Geometry check sheet. Reference: the model listing, model coordinates, mm. A direction names the side the tool comes from. Round coordinates to 2 decimals unless told otherwise and drop trailing zeros. Loops run counter-clockwise (first coordinate to the right, second up) from the corner with the lowest first, then second, coordinate; pieces in that order, holes last. Notation, with made-up numbers: (74, -35) -> (124, -35) arc R29 cw to (124, -11) -> close; hole circle Ø6 at (77, 71.25). An arc over 180 degrees is marked (long way). Use one line per item in the form item = value.
from build123d import *

# Parameters (mm, degrees)
BOSS_EXTRUDE1_DEPTH     = 12
CUT_EXTRUDE1_DEPTH      = 35.812889373272625
CUT_EXTRUDE1_DEPTH_BACK = 35.812889373272625
BOSS_EXTRUDE2_DEPTH     = 8
CUT_EXTRUDE2_DEPTH      = 2.5
CUT_EXTRUDE3_DEPTH      = 5
SKETCH8_R               = 1.4999999999999996
BOSS_EXTRUDE3_DEPTH     = 5.499999999999998
CUT_EXTRUDE4_DEPTH      = 35.812889373272625
CUT_EXTRUDE4_DEPTH_BACK = 35.812889373272625
SKETCH9_W               = 12
SKETCH9_H               = 6.684402113618233
CUT_EXTRUDE5_DEPTH      = 1


with BuildPart() as part:
    # Sketch1 → Boss-Extrude1 (new body)
    with BuildSketch(Plane.XY):
        with BuildLine():
            Line((-56.57427779976257, 0), (-40.22081023433309, 0))
            Line((-40.22081023433309, 0), (-41.713141903429594, 24.955419174788705))
            ThreePointArc((-41.713141903429594, 24.955419174788705), (-48.397544017047835, 31.639821288406946), (-55.081946130666076, 24.955419174788705))
            Line((-55.081946130666076, 24.955419174788705), (-56.57427779976257, 0))
        make_face()
    extrude(amount=BOSS_EXTRUDE1_DEPTH)

    # Sketch3 → Cut-Extrude1 (cut, two sides: drawn at the far end of the back side and taken through both)
    with BuildSketch(Plane(origin=(-48.39754401704783, 0, 0), x_dir=(0, 0, -1), z_dir=(1, 0, 0)).offset(-CUT_EXTRUDE1_DEPTH_BACK)):
        Polygon((-12, 6.613954943904592), (-12, 0), (-4, -4.9e-16), align=None)
    extrude(amount=CUT_EXTRUDE1_DEPTH + CUT_EXTRUDE1_DEPTH_BACK, mode=Mode.SUBTRACT)

    # Sketch6 → Boss-Extrude2 (add, symmetric)
    with BuildSketch(Plane(origin=(-48.39754401704783, 0, 0), x_dir=(0, 0, -1), z_dir=(1, 0, 0))):
        with BuildLine():
            ThreePointArc((-2.9999999999999982, -1.1000000000000008), (-3.0526985696936526, -0.5401658469562882), (-3.2089428526094457, 4.952e-14))
            Line((-3.2089428526094603, 0), (-4.98019609728148, 0))
            ThreePointArc((-4.980196097281471, 2.665e-14), (-4.62528078247269, -0.499877451714149), (-4.499999999999998, -1.1000000000000008))
            ThreePointArc((-4.499999999999998, -1.1000000000000012), (-6.600122548285821, -2.474719217527322), (-7.0198039027185715, -1.621e-14))
            Line((-7.019803902718577, 0), (-8.7910571473906, 0))
            ThreePointArc((-8.791057147390587, -4.152e-14), (-6.5598341530436635, -4.047301430306355), (-2.9999999999999982, -1.1000000000000014))
        make_face()
        with BuildLine():
            Line((-4.98019609728148, 0), (-3.2089428526094603, 0))
            ThreePointArc((-3.2089428526094457, 4.952e-14), (-6.000000000000047, 1.8999999999999992), (-8.791057147390587, -4.152e-14))
            Line((-8.7910571473906, 0), (-7.019803902718577, 0))
            ThreePointArc((-7.0198039027185715, -1.621e-14), (-6.00000000000003, 0.3999999999999988), (-4.980196097281471, 2.665e-14))
        make_face()
    extrude(amount=BOSS_EXTRUDE2_DEPTH, both=True)

    # Sketch6_3 → Cut-Extrude2 (cut, symmetric)
    with BuildSketch(Plane(origin=(-48.39754401704783, 0, 0), x_dir=(0, 0, -1), z_dir=(1, 0, 0))):
        with BuildLine():
            ThreePointArc((-2.9999999999999982, -1.1000000000000008), (-3.0526985696936526, -0.5401658469562882), (-3.2089428526094457, 4.952e-14))
            Line((-3.2089428526094603, 0), (-4.98019609728148, 0))
            ThreePointArc((-4.980196097281471, 2.665e-14), (-4.62528078247269, -0.499877451714149), (-4.499999999999998, -1.1000000000000008))
            ThreePointArc((-4.499999999999998, -1.1000000000000012), (-6.600122548285821, -2.474719217527322), (-7.0198039027185715, -1.621e-14))
            Line((-7.019803902718577, 0), (-8.7910571473906, 0))
            ThreePointArc((-8.791057147390587, -4.152e-14), (-6.5598341530436635, -4.047301430306355), (-2.9999999999999982, -1.1000000000000014))
        make_face()
        with BuildLine():
            Line((-4.98019609728148, 0), (-3.2089428526094603, 0))
            ThreePointArc((-3.2089428526094457, 4.952e-14), (-6.000000000000047, 1.8999999999999992), (-8.791057147390587, -4.152e-14))
            Line((-8.7910571473906, 0), (-7.019803902718577, 0))
            ThreePointArc((-7.0198039027185715, -1.621e-14), (-6.00000000000003, 0.3999999999999988), (-4.980196097281471, 2.665e-14))
        make_face()
    extrude(amount=CUT_EXTRUDE2_DEPTH, both=True, mode=Mode.SUBTRACT)

    # Sketch7 → Cut-Extrude3 (cut, symmetric)
    with BuildSketch(Plane(origin=(-48.39754401704783, 0, 0), x_dir=(0, 0, -1), z_dir=(1, 0, 0))):
        Polygon((-7.161655697006073, 2.6138810410171796), (-11.015220244212237, 5.799793827098392), (-7.829307458131025, 9.653358374304556), (-3.9757429109248625, 6.467445588223342), align=None)
    extrude(amount=CUT_EXTRUDE3_DEPTH, both=True, mode=Mode.SUBTRACT)

    # Sketch8 → Boss-Extrude3 (add, symmetric)
    with BuildSketch(Plane(origin=(-48.39754401704783, 0, 0), x_dir=(0, 0, -1), z_dir=(1, 0, 0))):
        with Locations((-7.548090255966457, 6.177113636233633)):
            Circle(SKETCH8_R)
    extrude(amount=BOSS_EXTRUDE3_DEPTH, both=True)

    # Sketch9 → Cut-Extrude4 (cut, two sides: drawn at the far end of the back side and taken through both)
    with BuildSketch(Plane(origin=(-48.39754401704783, 0, 0), x_dir=(0, 0, -1), z_dir=(1, 0, 0)).offset(-CUT_EXTRUDE4_DEPTH_BACK)):
        with Locations((-6, 28.297620231597822)):
            Rectangle(SKETCH9_W, SKETCH9_H)
    extrude(amount=CUT_EXTRUDE4_DEPTH + CUT_EXTRUDE4_DEPTH_BACK, mode=Mode.SUBTRACT)

    # Sketch10 → Cut-Extrude5 (cut, symmetric)
    with BuildSketch(Plane(origin=(-48.39754401704783, 0, 0), x_dir=(0, 0, -1), z_dir=(1, 0, 0))):
        Polygon((-2.32, -7.7e-16), (-0.31999999999999995, -1.1e-16), (-0.31999999999999995, 28.55038458807066), (-2.32, 28.55038458807066), align=None)
    extrude(amount=CUT_EXTRUDE5_DEPTH, both=True, mode=Mode.SUBTRACT)


solid = part.part
1. Gauge pin test, flat ends, axial feed: pin 1 (3.5 mm diameter, centred on y = -1.1, z = 6, fed in from +X); pin 2 (2 mm diameter, centred on y = 6, z = 7, fed in from +X); pin 3 (1 mm diameter, centred on y = 10.5, z = 1.5, fed in from +X); pin 4 (2.5 mm diameter, centred on y = -1.1, z = 6, fed in from -X) (3 decimals). Record the tip position at first contact, or that the pin passes through.
Return value:
pin_1 = -40.4
pin_2 = -40.52
pin_3 = -40.82
pin_4 = through
2. Mould release check, pull along X, two halves, no side actions. Record for faces 1 (the flat face through (-48, 13, 2.32)), 2 (the flat face through (-48, 24.955, 6)), 3 (the flat face through (-40.398, -2.4, 7.4)), 4 (the flat face through (-55.818, 12.652, 5.916)): released by +X, released by -X, zero draft, split by the parting line, or undercut.
Return value:
face_1 = undercut
face_2 = zero draft
face_3 = released by +X
face_4 = released by -X
3. Tool access check on faces 5 (the flat face through (-48.328, 8.083, 5.93)), 6 (the flat face through (-45.898, -2.4, 4.7)), 7 (the flat face through (-47.398, 13, 1)). Record the directions out of +Z, -Z, +X, -X, +Y, -Y that give a thin tool (end or side, any length) a straight path to the whole face; none if there is none.
Return value:
face_5 = none
face_6 = +Z, -Y
face_7 = +Y, -Y
4. Section check A-A (y = -1.1). Record the boundary of the cut face in (x, z).
Return value:
outline = (-56.4, 3) -> (-50.9, 3) -> (-50.9, 4.5) -> (-56.4, 4.5) -> close; (-56.4, 7.5) -> (-50.9, 7.5) -> (-50.9, 9) -> (-56.4, 9) -> close; (-45.9, 3) -> (-40.4, 3) -> (-40.4, 4.5) -> (-45.9, 4.5) -> close; (-45.9, 7.5) -> (-40.4, 7.5) -> (-40.4, 9) -> (-45.9, 9) -> close
5. Section check D-D (y = 3.5). Record the boundary of the cut face in (x, z).
Return value:
outline = (-56.36, 0) -> (-40.43, 0) -> (-40.43, 8.23) -> (-43.4, 8.23) -> (-43.4, 6.43) -> (-53.4, 6.43) -> (-53.4, 8.23) -> (-56.36, 8.23) -> close; hole (-49.4, 0.32) -> (-47.4, 0.32) -> (-47.4, 2.32) -> (-49.4, 2.32) -> close
6. Material ranges on line 1 along Y through (x, z) = (-55.05, 6); line 2 along Z through (x, y) = (-47.75, 23.25); line 3 along Z through (x, y) = (-54.8, -1.1), recorded low to high.
Return value:
line_1 = -4.1 to -2.6, 0.4 to 24.96
line_2 = 0 to 0.32, 2.32 to 12
line_3 = 3 to 4.5, 7.5 to 9
7. Section check C-C (x = -52). Record the boundary of the cut face in (y, z).
Return value:
outline = (0, 0) -> (24.96, 0) -> (24.96, 12) -> (6.61, 12) -> (5.8, 11.02) -> (9.65, 7.83) -> (6.47, 3.98) -> (2.61, 7.16) -> (1.89, 6.28) arc R3 ccw (long way) to (0, 3.21) -> close; circle Ø3 at (6.18, 7.55); hole circle Ø3 at (-1.1, 6)
8. Section check B-B (x = -48.5). Record the boundary of the cut face in (y, z), then the cut area to 3 significant figures.
Return value:
outline = (0, 0) -> (24.96, 0) -> (24.96, 0.32) -> (0, 0.32) -> close; (0, 2.32) -> (24.96, 2.32) -> (24.96, 12) -> (6.61, 12) -> (5.8, 11.02) -> (9.65, 7.83) -> (6.47, 3.98) -> (2.61, 7.16) -> (1.89, 6.28) arc R3 cw to (0, 3.21) -> close; circle Ø3 at (6.18, 7.55)
area = 203 mm2
